Answer from the drawing. Dimensions are ordinates in mm from the lowest x, y and z of the part. A direction names the side the tool comes from. Coordinates: 2 decimals unless noted, no trailing zeros. Order: outer loops, then holes, each group sorted by start corner. A loop starts at its lowest first (then second) coordinate and runs counter-clockwise, first axis right, second up. Notation, with made-up numbers: (68, -26.75) -> (107, -26.75) arc R27 cw to (107, -9.75) -> close; hole circle Ø5 at (50.25, 88.5). An arc over 180 degrees is marked (long way). Use CSV: the item, a comma, the result in double quotes.
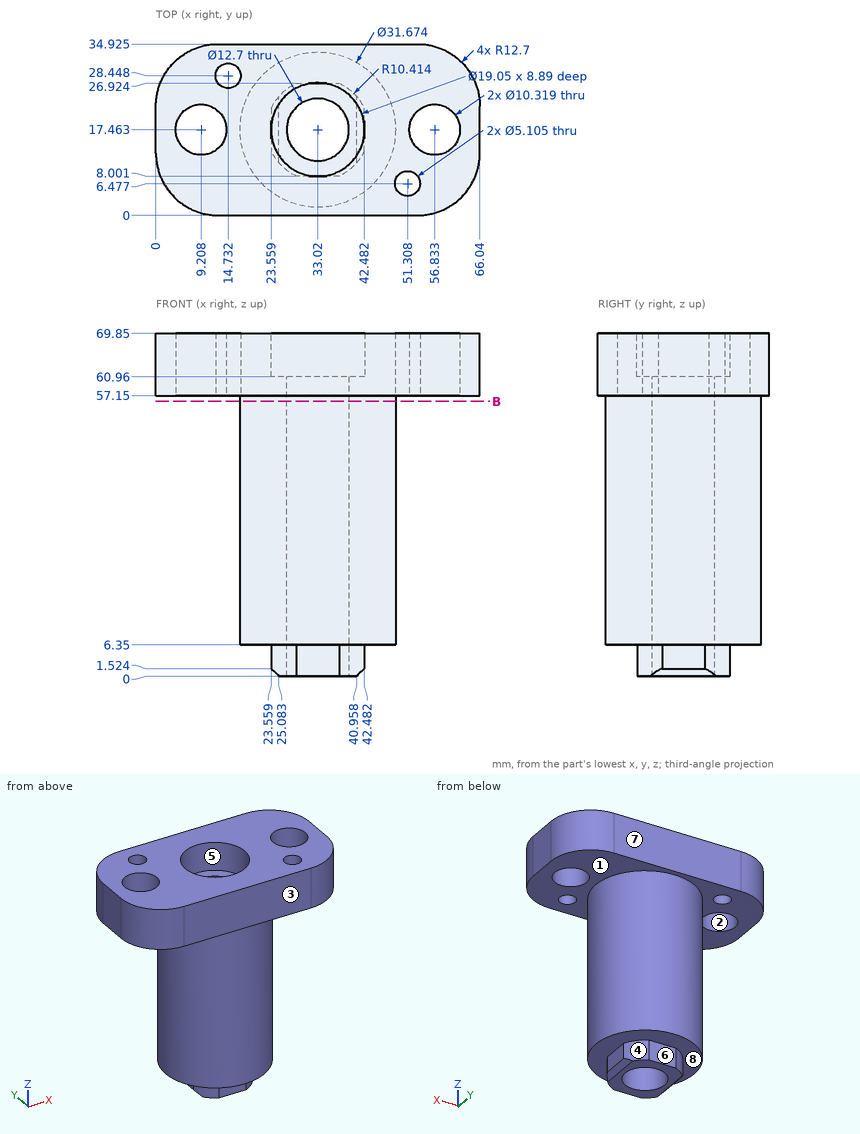
Item 1: Straight lines are drawn through the part: line 1 along X through (y, z) = (17.5, 62.5) (1 decimal); line 2 along Z through (x, y) = (47, 22.5); line 3 along Z through (x, y) = (22.5, 30.5). For each, find the intervals that lie inside material, in ascending order.
Return value:
line 1,"x = 0 to 4, 14.4 to 23.5, 42.5 to 51.7, 62 to 66"
line 2,"z = 6.35 to 69.85"
line 3,"z = 57.15 to 69.85"
Item 2: Find section B-B, the plane z = 56. Give the vertices of the cut face in (x, y).
Return value:
outline,"circle Ø31.67 at (33.02, 17.46); hole circle Ø12.7 at (33.02, 17.46)"
Item 3: The mould has two halves that part along Y. Classify the marked faces 1, 2 and 3: +Y half, -Y half, draft (parallel to the pull), parting line (faces both ways), or undercut.
Return value:
face 1,"draft"
face 2,"undercut"
face 3,"-Y half"
Item 4: Each of these flat-tipped pins is pushed along its axis until it touches: P1, Ø10, axis at y = 28, z = 16, coming from the +X side; P2, Ø1.5, axis at y = 30, z = 59, coming from the -X side; P3, Ø1.5, axis at x = 42, z = 41.5, coming from the +Y side. Where does it stop, or does it pass through?
Return value:
P1,"stops at x = 47.86"
P2,"stops at x = 2.12"
P3,"stops at y = 30.99"
Item 5: A tool of negligible diameter and unlimited length cuts with its end or side. For the marked faces 4, 5, 6, 7 and 8, from which of +Z, -Z, +X, -X, +Y, -Y can it reach the whole face along a straight path? Write none if from no direction.
Return value:
face 4,"-Z, +X, +Y"
face 5,"+Z"
face 6,"-Z, +X, -X, +Y"
face 7,"+Z, -Z, +X, -X, +Y"
face 8,"-Z"
